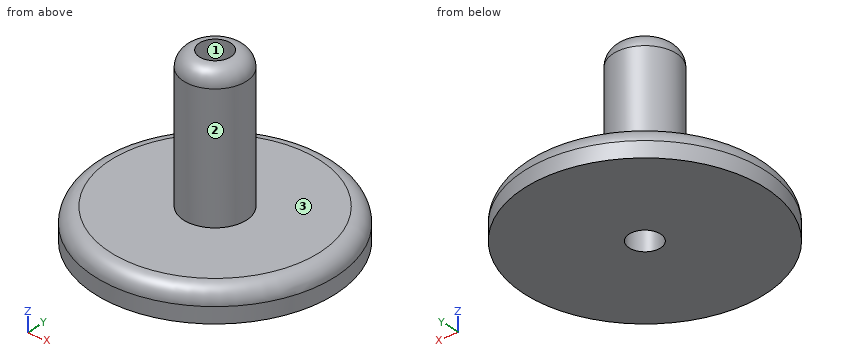
```python
from build123d import *

# Parameters (mm, degrees)
F0_R     = 7.6516982388
F0_R_2   = 1
F2_DEPTH = 2
F1_R     = 2
F1_R_2   = 1
F3_DEPTH = 9
F4_R     = 0.99999
F5_R     = 1


# Not quite as in the source:
# - a fillet or chamfer is up to 0.001 mm smaller than in the source, because OpenCascade refuses the exact size


with BuildPart() as f2:
    # F0 (on Top) → F2 (new body)
    with BuildSketch(Plane.XY):
        Circle(F0_R)
        Circle(F0_R_2, mode=Mode.SUBTRACT)
    extrude(amount=-F2_DEPTH)

    # F1 (on face) → F3 (join)
    with BuildSketch(Plane.XY):
        Circle(F1_R)
        Circle(F1_R_2, mode=Mode.SUBTRACT)
    extrude(amount=F3_DEPTH)

    # F4 (radius 1 in the source; OpenCascade refuses exactly that, so slightly less here)
    f4_edges = [f2.edges().sort_by_distance(p)[0] for p in [
        (-2, 0, 9),
    ]]
    fillet(f4_edges, radius=F4_R)

    # F5
    f5_edges = [f2.edges().sort_by_distance(p)[0] for p in [
        (-7.651698, 0, 0),
    ]]
    fillet(f5_edges, radius=F5_R)


solid = f2.part
```
Geometry check sheet. Reference: the model listing, model coordinates, mm. Face numbers are marked on the shaded views. Coordinates: 2 decimals unless noted, no trailing zeros. Order: outer loops, then holes, each group sorted by start corner. A loop starts at its lowest first (then second) coordinate and runs counter-clockwise, first axis right, second up. Notation, with made-up numbers: (52, 43.25) - (56, 43.25) arc R35 ccw to (56, 75.25) - close; hole circle Ø2 at (9.5, 65). An arc over 180 degrees is marked (long way). Use one line per item in the form item = value.
1. Section check C-C (z = 3.25). Record the boundary of the cut face in (x, y).
Here are the results:
outline = circle Ø4 at (0, 0); hole circle Ø2 at (0, 0)
2. Gauge pin test, flat ends, axial feed: pin 1 (4 mm diameter, centred on x = 2.5, z = 7.5, fed in from +Y); pin 2 (6 mm diameter, centred on x = 0.5, z = 5.5, fed in from -Y); pin 3 (2 mm diameter, centred on x = 3, y = 5, fed in from +Z). Record the tip position at first contact, or that the pin passes through.
Here are the results:
pin_1 = 1.94
pin_2 = -2
pin_3 = 0
3. Scan lines: line 1 (Y direction, x = 0, z = 4.5); line 2 (Z direction, x = -2.5, y = -4.75); line 3 (Y direction, x = -0.75, z = 6.75). Record each from-to range of solid material in increasing order.
Here are the results:
line_1 = -2 to -1, 1 to 2
line_2 = -2 to 0
line_3 = -1.85 to -0.66, 0.66 to 1.85
4. Draft check along Y on the marked faces 1, 2 and 3. Enter one of: pulls with the +Y half, pulls with the -Y half, needs draft (parallel to the pull), parting line crosses it, or undercut.
Here are the results:
face_1 = undercut
face_2 = parting line crosses it
face_3 = needs draft
